Part model, mm, in its own coordinate system. A direction names the side the tool comes from. Coordinates: 2 decimals unless noted, no trailing zeros. Order: outer loops, then holes, each group sorted by start corner. A loop starts at its lowest first (then second) coordinate and runs counter-clockwise, first axis right, second up.
Autodesk Inventor part; units mm, degrees
ref_plane "YZ Plane" through (0, 0, 0) normal (1, 0, 0) x (0, 1, 0)
ref_plane "XZ Plane" through (0, 0, 0) normal (0, 1, 0) x (-1, 0, 0)
ref_plane "XY Plane" through (0, 0, 0) normal (0, 0, 1) x (1, 0, 0)
sketch "Sketch1" plane through (0, 0, 0) normal (0, 0, 1) x (1, 0, 0)
  line L0 (-1.96, -1.4194) -> (1.96, -1.4194)
  line L1 (1.96, 1.4194) -> (-1.96, 1.4194)
  arc A0 (-1.96, 1.4194) -> (-1.96, -1.4194) centre (0, 0) ccw
  arc A1 (1.96, -1.4194) -> (1.96, 1.4194) centre (0, 0) ccw
  line L2 (-7.5, -7.5) -> (7.5, -7.5)
  line L3 (7.5, -7.5) -> (7.5, 7.5)
  line L4 (7.5, 7.5) -> (-7.5, 7.5)
  line L5 (-7.5, 7.5) -> (-7.5, -7.5)
  line L6 (-7.5, -7.5) -> (7.5, 7.5) construction
  line L7 (7.5, -7.5) -> (-7.5, 7.5) construction
  line L8 (-5.5, 2.58) -> (-2.66, 2.58)
  line L9 (-2.66, 2.58) -> (-2.66, 5.5)
  line L10 (-2.66, 5.5) -> (-5.5, 5.5)
  line L11 (-5.5, 5.5) -> (-5.5, 2.58)
  line L12 (0, 0) -> (0, 4.08) construction
  line L13 (0, 0) -> (5.4269, 0) construction
  line L14 (5.5, 2.58) -> (2.66, 2.58)
  line L15 (2.66, 2.58) -> (2.66, 5.5)
  line L16 (2.66, 5.5) -> (5.5, 5.5)
  line L17 (5.5, 5.5) -> (5.5, 2.58)
  line L18 (-5.5, -2.58) -> (-2.66, -2.58)
  line L19 (-2.66, -2.58) -> (-2.66, -5.5)
  line L20 (-2.66, -5.5) -> (-5.5, -5.5)
  line L21 (-5.5, -5.5) -> (-5.5, -2.58)
  line L22 (2.66, -2.58) -> (2.66, -5.5)
  line L23 (2.66, -5.5) -> (5.5, -5.5)
  line L24 (5.5, -5.5) -> (5.5, -2.58)
  line L25 (5.5, -2.58) -> (2.66, -2.58)
  point P0 (0, -4.08)
  dimension "d3" = 3.92
  dimension "d4" = 2.42
  dimension "d5" = 15
  dimension "d7" = 2.84
  dimension "d8" = 2.92
  dimension "d9" = 2
  dimension "d10" = 2
extrude "Extrusion1" add sketch "Sketch1" along normal blind 3
properties part number "motor_bottom"
Q1. Wall check: line 1 along Y through (x, z) = (4.25, 0.95); line 2 along X through (y, z) = (-3.75, 1.7); line 3 along Y through (x, z) = (1.5, 2.45). Give the ranges that are in metal, low to high.
Results list:
line 1: y = -7.5 to -5.5, -2.58 to 2.58, 5.5 to 7.5
line 2: x = -7.5 to -5.5, -2.66 to 2.66, 5.5 to 7.5
line 3: y = -7.5 to -1.42, 1.42 to 7.5
Q2. Cut at D-D on y = 0.5. Write the cut outline in (x, z), and give its area (3 significant figures).
Results list:
outline: (-7.5, 0) - (-2.37, 0) - (-2.37, 3) - (-7.5, 3) - close; (2.37, 0) - (7.5, 0) - (7.5, 3) - (2.37, 3) - close
area: 30.8 mm2
Q3. Which spindle directions (+Z, -Z, +X, -X, +Y, -Y) get a long thin tool onto all of the face, cutting with end or side? Do faces 4 (the face through (4, 5.5, 1)), 5 (the face through (0, 2, 3)). Say none if no direction does.
Results list:
face 4: +Z, -Z
face 5: +Z, +X, -X, +Y, -Y
Q4. Cut at C-C on z = 0.7. Write the cut outline in (x, y).
Results list:
outline: (-7.5, -7.5) - (7.5, -7.5) - (7.5, 7.5) - (-7.5, 7.5) - close; hole (-5.5, -5.5) - (-2.66, -5.5) - (-2.66, -2.58) - (-5.5, -2.58) - close; hole (-5.5, 2.58) - (-2.66, 2.58) - (-2.66, 5.5) - (-5.5, 5.5) - close; hole (-1.96, -1.42) - (1.96, -1.42) arc R2.42 ccw to (1.96, 1.42) - (-1.96, 1.42) arc R2.42 ccw to start; hole (2.66, -5.5) - (5.5, -5.5) - (5.5, -2.58) - (2.66, -2.58) - close; hole (2.66, 2.58) - (5.5, 2.58) - (5.5, 5.5) - (2.66, 5.5) - close
Q5. Pin check, flat tip, straight feed: pin 1 Ø1 at (x, y) = (-3, 2) entering from -Z. Stop position of the tip, or through.
Results list:
pin 1: stops at z = 0
Q6. Cut at B-B on x = -5. Write the cut outline in (y, z), and give its area (3 significant figures).
Results list:
outline: (-7.5, 0) - (-5.5, 0) - (-5.5, 3) - (-7.5, 3) - close; (-2.58, 0) - (2.58, 0) - (2.58, 3) - (-2.58, 3) - close; (5.5, 0) - (7.5, 0) - (7.5, 3) - (5.5, 3) - close
area: 27.5 mm2
Q7. Cut at A-A on y = -5. Write the cut outline in (x, z), and give its area (3 significant figures).
Results list:
outline: (-7.5, 0) - (-5.5, 0) - (-5.5, 3) - (-7.5, 3) - close; (-2.66, 0) - (2.66, 0) - (2.66, 3) - (-2.66, 3) - close; (5.5, 0) - (7.5, 0) - (7.5, 3) - (5.5, 3) - close
area: 28.0 mm2
Q8. Mould opens along Y. For faces 1 (the face through (0, 7.5, 1)), 2 (the face through (0, -7.5, 1)), 3 (the face through (-4, 5.5, 1)) say: pulls with the +Y half, pulls with the -Y half, needs draft (parallel to the pull), parting line crosses it, or undercut.
Results list:
face 1: pulls with the +Y half
face 2: pulls with the -Y half
face 3: undercut
